```python
from build123d import *

# Parameters (mm, degrees)
F0_R     = 1.375
F0_W     = 7
F0_H     = 3.2
F0_W_2   = 3.2
F0_H_2   = 13
F1_DEPTH = 1.5


with BuildPart() as f1:
    # F0 (on Top) → F1 (new body, symmetric)
    with BuildSketch(Plane.XY):
        with BuildLine():
            Line((-27.8, -32.5), (27.8, -32.5))
            Line((27.8, -32.5), (27.8, -19.5))
            Line((27.8, -19.5), (31, -19.5))
            Line((31, -19.5), (35.796361, -19.5))
            ThreePointArc((35.796361, -19.5), (41.42, 0), (35.796361, 19.5))
            Line((35.796361, 19.5), (31, 19.5))
            Line((31, 19.5), (27.8, 19.5))
            Line((27.8, 19.5), (27.8, 32.5))
            Line((27.8, 32.5), (-27.8, 32.5))
            Line((-27.8, 32.5), (-27.8, 19.5))
            Line((-27.8, 19.5), (-31, 19.5))
            Line((-31, 19.5), (-31, 6.5))
            Line((-31, 6.5), (-27.8, 6.5))
            Line((-27.8, 6.5), (-27.8, -6.5))
            Line((-27.8, -6.5), (-31, -6.5))
            Line((-31, -6.5), (-31, -19.5))
            Line((-31, -19.5), (-27.8, -19.5))
            Line((-27.8, -19.5), (-27.8, -32.5))
        make_face()
        with Locations((-24.5, -29)):
            Circle(F0_R, mode=Mode.SUBTRACT)
        with Locations((-6.5, -25.9)):
            Rectangle(F0_W, F0_H, mode=Mode.SUBTRACT)
        with Locations((6.5, -25.9)):
            Rectangle(F0_W, F0_H, mode=Mode.SUBTRACT)
        with Locations((24.5, -29)):
            Circle(F0_R, mode=Mode.SUBTRACT)
        with Locations((34.2, -13)):
            Rectangle(F0_W_2, F0_H, mode=Mode.SUBTRACT)
        with Locations((-24.5, 29)):
            Circle(F0_R, mode=Mode.SUBTRACT)
        with Locations((29.4, 0)):
            Rectangle(F0_W_2, F0_H_2, mode=Mode.SUBTRACT)
        Polygon((32.6, 1.6), (34.2, 1.6), (35.8, 1.6), (35.8, -1.6), (32.6, -1.6), align=None, mode=Mode.SUBTRACT)
        with Locations((34.2, 13)):
            Rectangle(F0_W_2, F0_H, mode=Mode.SUBTRACT)
        with Locations((24.5, 29)):
            Circle(F0_R, mode=Mode.SUBTRACT)
    extrude(amount=F1_DEPTH, both=True)


solid = f1.part
```
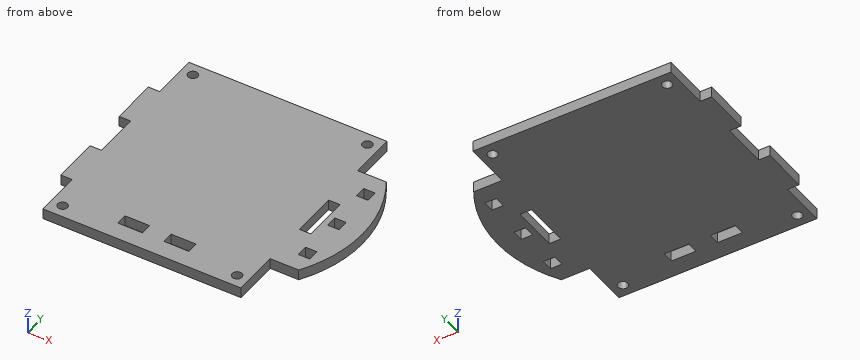
The model under review builds one solid part; all positions refer to its coordinate system, in mm. Give positions to 0.01 mm unless a question says otherwise; leave off trailing zeros. Write each loop counter-clockwise with the first axis right and the second up, starting at its lowest first coordinate (ties: lowest second). Pieces come first, ordered by that corner, then holes. Notation, with made-up numbers: (47, 64) -> (85, 64) arc R38 ccw to (85, 103) -> close; hole circle Ø11 at (16, 16.5). An arc over 180 degrees is marked (long way). Answer in a Markdown table with one row per item.
1) Clearance check with flat-ended pins moving along their axes: P1, Ø1.5, axis at x = 30, z = 0.5, coming from the -Y side; P2, Ø0.9, axis at x = 29.5, z = -0.5, coming from the +Y side; P3, Ø1.5, axis at y = 0.5, z = -0.5, coming from the -X side; P4, Ø1.6, axis at x = 24.5, y = -29, coming from the -Z side. State where each tip first meets the part, or that it passes through.
Worked answers:
| item | result |
|---|---|
| P1 | y = -19.5 |
| P2 | y = 19.5 |
| P3 | x = -27.8 |
| P4 | through |
2) For L1, parallel to Y at x = 24.5, z = 0.9 (3 decimals); L2, parallel to Y at x = -7.5, z = -1.4; L3, parallel to Y at x = -23.5, z = -1.3, list the stretches that pass through material, from the lowest coordinate up. Write a range as [from, to].
Worked answers:
| item | result |
|---|---|
| L1 | [-32.5, -30.375], [-27.625, 27.625], [30.375, 32.5] |
| L2 | [-32.5, -27.5], [-24.3, 32.5] |
| L3 | [-32.5, -29.94], [-28.06, 28.06], [29.94, 32.5] |
3) Add section A-A on y = -25.5. State the section outline as (x, z) points, plus the area to 3 significant figures.
Worked answers:
| item | result |
|---|---|
| outline | (-27.8, -1.5) -> (-10, -1.5) -> (-10, 1.5) -> (-27.8, 1.5) -> close; (-3, -1.5) -> (3, -1.5) -> (3, 1.5) -> (-3, 1.5) -> close; (10, -1.5) -> (27.8, -1.5) -> (27.8, 1.5) -> (10, 1.5) -> close |
| area | 125 mm² |
4) Add section C-C on x = -24.5. State the section outline as (y, z) points (3 decimals), plus the area to 4 significant figures.
Worked answers:
| item | result |
|---|---|
| outline | (-32.5, -1.5) -> (-30.375, -1.5) -> (-30.375, 1.5) -> (-32.5, 1.5) -> close; (-27.625, -1.5) -> (27.625, -1.5) -> (27.625, 1.5) -> (-27.625, 1.5) -> close; (30.375, -1.5) -> (32.5, -1.5) -> (32.5, 1.5) -> (30.375, 1.5) -> close |
| area | 178.5 mm² |
5) Add section B-B on x = 33.5. State the section outline as (y, z) points, plus the area to 3 significant figures.
Worked answers:
| item | result |
|---|---|
| outline | (-19.5, -1.5) -> (-14.6, -1.5) -> (-14.6, 1.5) -> (-19.5, 1.5) -> close; (-11.4, -1.5) -> (-1.6, -1.5) -> (-1.6, 1.5) -> (-11.4, 1.5) -> close; (1.6, -1.5) -> (11.4, -1.5) -> (11.4, 1.5) -> (1.6, 1.5) -> close; (14.6, -1.5) -> (19.5, -1.5) -> (19.5, 1.5) -> (14.6, 1.5) -> close |
| area | 88.2 mm² |
6) Add section D-D on x = 6. State the section outline as (y, z) points.
Worked answers:
| item | result |
|---|---|
| outline | (-32.5, -1.5) -> (-27.5, -1.5) -> (-27.5, 1.5) -> (-32.5, 1.5) -> close; (-24.3, -1.5) -> (32.5, -1.5) -> (32.5, 1.5) -> (-24.3, 1.5) -> close |
